Autodesk Inventor part; units mm, degrees
ref_plane "YZ Plane" through (0, 0, 0) normal (1, 0, 0) x (0, 1, 0)
ref_plane "XZ Plane" through (0, 0, 0) normal (0, 1, 0) x (-1, 0, 0)
ref_plane "XY Plane" through (0, 0, 0) normal (0, 0, 1) x (1, 0, 0)
sketch "Sketch1" plane through (0, 0, 0) normal (0, 1, 0) x (-1, 0, 0)
  line L0 (-90, 75) -> (90, 75)
  line L1 (90, 75) -> (90, -75)
  line L2 (90, -75) -> (-90, -75)
  line L3 (-90, -75) -> (-90, 75)
  line L4 (-90, 75) -> (90, -75) construction
  line L5 (90, 75) -> (-90, -75) construction
  point P0 (0, 0)
  dimension "d0" = 180
  dimension "d1" = 150
extrude "Extrusion1" add sketch "Sketch1" along normal blind 3
offset faces "Size1" outward 0.5 faces at (-30, 1, 75) (30, 1, -75)
sketch "Sketch2" plane through (0, 0, 0) normal (0, -1, 0) x (1, 0, 0)
  line L0 (-90, -75.5) -> (-90, 75.5)
  line L1 (-90, 20) -> (-85, 20)
  line L2 (-85, 20) -> (-85, -20)
  line L3 (-85, -20) -> (-90, -20)
  line L4 (-90, -20) -> (-90, 20)
  point P0 (0, 0)
  point P1 (-90, -77.5)
  point P2 (-90, 77.5)
  point P3 (-85, 0)
  point P4 (-90, 0)
  dimension "d6" = 40
  dimension "d7" = 5
extrude "Extrusion2" cut sketch "Sketch2" against normal blind 10
sketch "Sketch3" plane through (0, 0, 0) normal (0, -1, 0) x (1, 0, 0)
  circle A0 centre (75, 60) radius 2.4
  circle A1 centre (75, 0) radius 2.4
  circle A2 centre (75, -60) radius 2.4
  circle A3 centre (-75, 60) radius 2.4
  circle A4 centre (-75, 0) radius 2.4
  circle A5 centre (-75, -57.6) radius 2.4
  point P0 (0, 0)
  dimension "d10" = 4.8
extrude "Extrusion3" cut sketch "Sketch3" against normal blind 10
properties part number "Front plane" material "Wood (Birch)"
Here's how the part is built. I have some questions about the finished solid (model axes, mm). Coordinates: 2 decimals unless noted, no trailing zeros. Order: outer loops, then holes, each group sorted by start corner. A loop starts at its lowest first (then second) coordinate and runs counter-clockwise, first axis right, second up. Notation, with made-up numbers: M -5,66.5 L 53,66.5 A23 cw 53,94.5 Z; hole C -17,-18.5 d11. An arc over 180 degrees is marked long. Answer as a JSON object with one key per item and string values. Group by question number.
(1) Suppose I cut it at A-A, the plane z = 60. Please give me the cut outline in (x, y), then the cut area to 3 significant figures.
(2) Suppose I cut it at C-C, the plane z = 0. Please give me the cut outline in (x, y), then the cut area to 3 significant figures.
(3) If we mould it in two halves opening along X, with no side actions, what happens to faces 1 (the face through (77.29, 1.48, 60.72)), 2 (the face through (1, 3, 1))? For each: released by +X, released by -X, zero draft, split by the parting line, or undercut.
(4) I need wall thicknesses on probe 1 along Z at (x, y) = (-75, 2.4); probe 2 along X at (y, z) = (2.3, 60.5); probe 3 along X at (y, z) = (0.2, 3). Which ranges of each line are inside material? Lowest first, please.
(5) Suppose I cut it at B-B, the plane x = -75. Please give me the cut outline in (y, z), then the cut area to 3 significant figures.
Values found:
{
 "1": {"outline": "M -90,0 L -77.4,0 L -77.4,3 L -90,3 Z; M -72.6,0 L 72.6,0 L 72.6,3 L -72.6,3 Z; M 77.4,0 L 90,0 L 90,3 L 77.4,3 Z", "area": "511 mm^2"},
 "2": {"outline": "M -85,0 L -77.4,0 L -77.4,3 L -85,3 Z; M -72.6,0 L 72.6,0 L 72.6,3 L -72.6,3 Z; M 77.4,0 L 90,0 L 90,3 L 77.4,3 Z", "area": "496 mm^2"},
 "3": {"face 1": "undercut", "face 2": "zero draft"},
 "4": {"probe 1": "z = -75.5 to -60, -55.2 to -2.4, 2.4 to 57.6, 62.4 to 75.5", "probe 2": "x = -90 to -77.35, -72.65 to 72.65, 77.35 to 90", "probe 3": "x = -85 to 90"},
 "5": {"outline": "M 0,-75.5 L 3,-75.5 L 3,-60 L 0,-60 Z; M 0,-55.2 L 3,-55.2 L 3,-2.4 L 0,-2.4 Z; M 0,2.4 L 3,2.4 L 3,57.6 L 0,57.6 Z; M 0,62.4 L 3,62.4 L 3,75.5 L 0,75.5 Z", "area": "410 mm^2"}
}
